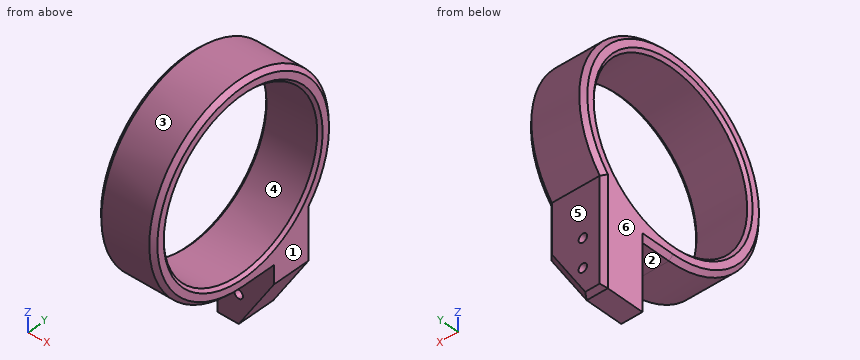
```python
from build123d import *

# Parameters (mm, degrees)
SKETCH_1_R          = 35
EXTRUDE_1_DEPTH     = 20
SKETCH_2_R          = 30
CUT_EXTRUDE_1_DEPTH = 54.38539126
SKETCH_3_W          = 20
SKETCH_3_H          = 15
EXTRUDE_2_DEPTH     = 25
EXTRUDE_3_REACH     = 82.777
SKETCH_4_W          = 20
SKETCH_4_H          = 12
SKETCH_5_R          = 30
CUT_EXTRUDE_2_DEPTH = 73.284161474
CUT_EXTRUDE_3_REACH = 90.566
SKETCH_8_R          = 1.5
CUT_EXTRUDE_4_DEPTH = 79.797208072
CHAMFER_1_SIZE      = 1
CHAMFER_2_SIZE      = 1.5


with BuildPart() as part:
    # 草图1 → 凸台-拉伸1 (new body)
    with BuildSketch(Plane(origin=(0, 0, 0), x_dir=(0, 0, -1), z_dir=(1, 0, 0))):
        Circle(SKETCH_1_R)
    extrude(amount=EXTRUDE_1_DEPTH)

    # 草图2 → 切除-拉伸1 (cut, through all)
    with BuildSketch(Plane(origin=(20, 0, 0), x_dir=(0, 0, -1), z_dir=(1, 0, 0))):
        Circle(SKETCH_2_R)
    extrude(amount=-CUT_EXTRUDE_1_DEPTH, mode=Mode.SUBTRACT)

    # 草图3 → 凸台-拉伸2 (add, symmetric)
    with BuildSketch(Plane(origin=(0, 0, -35), x_dir=(-1, 0, 0), z_dir=(0, 0, -1))):
        with Locations((-10, 19.5)):
            Rectangle(SKETCH_3_W, SKETCH_3_H)
    extrude(amount=EXTRUDE_2_DEPTH, both=True)

    # 草图4 → 凸台-拉伸3 (add, up to next)
    with BuildSketch(Plane(origin=(0, 0, -35), x_dir=(-1, 0, 0), z_dir=(0, 0, -1)), mode=Mode.PRIVATE) as extrude_3_sk1:
        with Locations((-10, 6)):
            Rectangle(SKETCH_4_W, SKETCH_4_H)
    extrude_3_tool1 = extrude(extrude_3_sk1.sketch, amount=-EXTRUDE_3_REACH, mode=Mode.PRIVATE) - part.part
    add(extrude_3_tool1.solids().sort_by_distance((10, 6, -35))[0])

    # 草图5 → 切除-拉伸2 (cut, through all)
    with BuildSketch(Plane(origin=(20, 0, 0), x_dir=(0, 0, -1), z_dir=(1, 0, 0))):
        Circle(SKETCH_5_R)
    extrude(amount=-CUT_EXTRUDE_2_DEPTH, mode=Mode.SUBTRACT)

    # 草图6 → 切除-拉伸3 (cut, up to next)
    with BuildSketch(Plane(origin=(0, 27, 0), x_dir=(1, 0, 0), z_dir=(0, 1, 0)), mode=Mode.PRIVATE) as cut_extrude_3_sk1:
        Polygon((7.5, 60), (20, 40), (20, 60), align=None)
    cut_extrude_3_tool1 = extrude(cut_extrude_3_sk1.sketch, amount=-CUT_EXTRUDE_3_REACH, mode=Mode.PRIVATE) & part.part
    add(cut_extrude_3_tool1.solids().sort_by_distance((15.833333, 27, -53.333333))[0], mode=Mode.SUBTRACT)

    # 草图8 → 切除-拉伸4 (cut, through all)
    with BuildSketch(Plane(origin=(0, 12, 0), x_dir=(-1, 0, 0), z_dir=(0, -1, 0))):
        with Locations(Location((-7.5, 40, 0), (0, 0, 180))):
            Circle(SKETCH_8_R)
        with Locations(Location((-7.5, 50, 0), (0, 0, 180))):
            Circle(SKETCH_8_R)
    extrude(amount=-CUT_EXTRUDE_4_DEPTH, mode=Mode.SUBTRACT)

    # 倒角1
    chamfer_1_edges = [part.edges().sort_by_distance(p)[0] for p in [
        (0, -12, 27.49545417),
        (20, -12, 27.49545417),
    ]]
    chamfer(chamfer_1_edges, length=CHAMFER_1_SIZE)

    # 倒角2
    chamfer_2_edges = [part.edges().sort_by_distance(p)[0] for p in [
        (0, -14.925029132, 31.658229663),
        (20, -14.925029132, 31.658229663),
        (0, 27, -41.135528726),
        (3.75, 27, -60),
        (20, 6, -35),
        (0, 6, -35),
        (20, 27, -31.135528726),
        (13.75, 27, -50),
    ]]
    chamfer(chamfer_2_edges, length=CHAMFER_2_SIZE)


solid = part.part
```
Read the model definition and answer for the solid it produces. Units are mm, in the model's axes. Face numbers are marked on the shaded views. A direction names the side the tool comes from. Round coordinates to 2 decimals unless told otherwise and drop trailing zeros. Write each loop counter-clockwise with the first axis right and the second up, starting at its lowest first coordinate (ties: lowest second). Pieces come first, ordered by that corner, then holes. Notation, with made-up numbers: (15.25, 46.25) - (69.25, 46.25) arc R24 ccw to (69.25, 61.25) - close; hole circle Ø6 at (48.5, 32.5). An arc over 180 degrees is marked (long way). One line per item, written item: value.
Q1. Which of the six approach directions +Z, -Z, +X, -X, +Y, -Y give full straight-line access (tool end or side, diameter ignored) to the marked faces 5 and 6?
The answers:
face 5: -Z, +X, -X, +Y
face 6: +Z, -Z, -X, +Y, -Y
Q2. Each of these flat-tipped pins is pushed along its axis until it touches: P1, Ø5, axis at x = 9.5, y = -13.5, coming from the +Z side; P2, Ø8, axis at x = 15.5, z = -22.5, coming from the -Y side; P3, Ø1, axis at x = 16, z = 3, coming from the +Y side. Where does it stop, or does it pass through?
The answers:
P1: stops at z = 33.23
P2: stops at y = -29.71
P3: stops at y = 34.91
Q3. Find section B-B (y = 14.5). Count the separate pieces of the cut face and the enclosed holes in it, and give its area (3 significant figures).
The answers:
separate pieces: 2
enclosed holes: 2
area: 643 mm2
Q4. Straight lines are drawn through the part: line 1 (Y direction, x = 9.5, z = 0); line 2 (Z direction, x = 7.5, y = 21.75); line 3 (Z direction, x = 7.5, y = 19). For each, find the intervals that lie inside material, in ascending order. Write a range as from..to.
The answers:
line 1: y = -35..-30, 30..35
line 2: z = -60..-51.5, -48.5..-41.5, -38.5..-20.66, 20.66..27.42
line 3: z = -60..-51.5, -48.5..-41.5, -38.5..-23.22, 23.22..29.39
Q5. For a pull along Z with two mould halves and no side action, classify the marked faces 1, 2, 3 and 4 as pulls with the +Z half, pulls with the -Z half, needs draft (parallel to the pull), parting line crosses it, or undercut.
The answers:
face 1: needs draft
face 2: pulls with the -Z half
face 3: parting line crosses it
face 4: undercut
Q6. Find section A-A (x = 10). Determine the outline of the cut face in (y, z), and give its area (3 significant figures).
The answers:
outline: (0, -35) - (12, -35) - (12, -56) - (25.5, -56) - (27, -53.17) - (27, -22.27) arc R35 ccw (long way) to start; hole circle Ø60 at (0, 0)
area: 1,440 mm2
